from build123d import *

# Parameters (mm, degrees)
SKETCH1_R           = 57.15
SKETCH1_R_2         = 50.8
BOSS_EXTRUDE1_DEPTH = 177.8
SKETCH3_R           = 1.5875
CUT_EXTRUDE1_DEPTH  = 6.35
CIRPATTERN1_COUNT   = 8


with BuildPart() as part:
    # Sketch1 → Boss-Extrude1 (new body)
    with BuildSketch(Plane(origin=(0, 0, 0), x_dir=(1, 0, 0), z_dir=(0, 1, 0))):
        Circle(SKETCH1_R)
        Circle(SKETCH1_R_2, mode=Mode.SUBTRACT)
    extrude(amount=BOSS_EXTRUDE1_DEPTH)

    # Sketch3 → Cut-Extrude1 (cut, symmetric)
    with BuildSketch(Plane.XY.offset(53.975)):
        with Locations((0, 127)):
            Circle(SKETCH3_R)
    cut_extrude1 = extrude(amount=CUT_EXTRUDE1_DEPTH, both=True, mode=Mode.SUBTRACT)

    # CirPattern1: Cut-Extrude1 ×8 about axis
    cirpattern1_axis = Axis((0, 177.8, 0), (0, 1, 0))
    for i in range(1, CIRPATTERN1_COUNT):
        add(cut_extrude1.rotate(cirpattern1_axis, i * 360 / CIRPATTERN1_COUNT), mode=Mode.SUBTRACT)


solid = part.part
The listing builds one solid part. Answer for the finished solid, in the listing's coordinates (mm). Give positions to 0.01 mm unless a question says otherwise; leave off trailing zeros. Order: outer loops, then holes, each group sorted by start corner. A loop starts at its lowest first (then second) coordinate and runs counter-clockwise, first axis right, second up. Notation, with made-up numbers: (-17, 17.25) -> (7, 17.25) arc R27 ccw to (7, 41.25) -> close; hole circle Ø10 at (4.25, 42.5). An arc over 180 degrees is marked (long way). Put each result on its own line as item: value.
Item 1: A cutting plane is placed at C-C on y = 72.5. Give the vertices of the cut face in (x, z), plus the area to 3 significant figures.
Established:
outline: circle Ø114.3 at (0, 0); hole circle Ø101.6 at (0, 0)
area: 2,150 mm^2
Item 2: Given P1, Ø2, axis at x = -12.5, y = 148.5, coming from the -Z side; P2, Ø2.5, axis at x = 0, y = 127, coming from the -Z side; P3, Ø12, axis at y = 44.5, z = -27.5, coming from the +X side; P4, Ø5, axis at y = 127, z = 0, coming from the +X side, each flat-ended and moving along its own axis, determine where each tip first touches the part or whether it passes through.
Established:
P1: stops at z = -55.98
P2: passes through
P3: stops at x = 52.95
P4: stops at x = 57.15
Item 3: For a pull along X with two mould halves and no side action, classify faces 1 (the face through (37.95, 125.45, 38.43)), 2 (the face through (-38, 177.8, 34)), 3 (the face through (-37.95, 125.45, -38.43)), 4 (the face through (-57.095, 87.655, -2.513)) as released by +X, released by -X, zero draft, split by the parting line, or undercut.
Established:
face 1: undercut
face 2: zero draft
face 3: undercut
face 4: split by the parting line
Item 4: A cutting plane is placed at B-B on x = 7. Give the vertices of the cut face in (y, z).
Established:
outline: (0, -56.72) -> (177.8, -56.72) -> (177.8, -50.32) -> (0, -50.32) -> close; (0, 50.32) -> (177.8, 50.32) -> (177.8, 56.72) -> (0, 56.72) -> close
Item 5: Straight lines are drawn through the part: line 1 (Z direction, x = 0, y = 40); line 2 (Z direction, x = -32.5, y = 21). For each, find the intervals that lie inside material, in ascending order.
Established:
line 1: z = -57.15 to -50.8, 50.8 to 57.15
line 2: z = -47.01 to -39.04, 39.04 to 47.01
Item 6: A cutting plane is placed at A-A on z = 45.5. Give the vertices of the cut face in (x, y).
Established:
outline: (-34.58, 0) -> (-22.59, 0) -> (-22.59, 177.8) -> (-34.58, 177.8) -> close; (22.59, 0) -> (34.58, 0) -> (34.58, 177.8) -> (22.59, 177.8) -> close
